Work out the finished part from the listing and answer in its coordinate system (mm). A direction names the side the tool comes from. Coordinates: 2 decimals unless noted, no trailing zeros. Loops run counter-clockwise (first coordinate to the right, second up) from the corner with the lowest first, then second, coordinate; pieces in that order, holes last. Notation, with made-up numbers: (-9.5, 84) -> (4.5, 84) arc R31 cw to (4.5, 115) -> close; hole circle Ø8 at (-4, 51). An arc over 180 degrees is marked (long way). Use a Markdown table: item, result.
from build123d import *

# Parameters (mm, degrees)
SKETCH1_R           = 21.25
SKETCH1_R_2         = 1.5
BOSS_EXTRUDE1_DEPTH = 5
CHAMFER1_SIZE       = 2.5
SKETCH2_R           = 4.75
BOSS_EXTRUDE2_DEPTH = 2


with BuildPart() as part:
    # Sketch1 → Boss-Extrude1 (new body)
    with BuildSketch(Plane(origin=(0, 0, 0), x_dir=(1, 0, 0), z_dir=(0, 1, 0))):
        with Locations(Location((0, 0, 0), (0, 0, 270))):
            Circle(SKETCH1_R)
        with Locations(Location((0, 15.5, 0), (0, 0, 270))):
            Circle(SKETCH1_R_2, mode=Mode.SUBTRACT)
        with Locations(Location((15.5, 0, 0), (0, 0, 270))):
            Circle(SKETCH1_R_2, mode=Mode.SUBTRACT)
        with Locations(Location((0, -15.5, 0), (0, 0, 270))):
            Circle(SKETCH1_R_2, mode=Mode.SUBTRACT)
        with Locations(Location((-15.5, 0, 0), (0, 0, 270))):
            Circle(SKETCH1_R_2, mode=Mode.SUBTRACT)
        with BuildLine():
            Line((-1.532970972, 2.1), (1.532970972, 2.1))
            ThreePointArc((1.532970972, 2.1), (0, -2.6), (-1.532970972, 2.1))
        make_face(mode=Mode.SUBTRACT)
    extrude(amount=BOSS_EXTRUDE1_DEPTH)

    # Chamfer1
    chamfer1_edges = [part.edges().sort_by_distance(p)[0] for p in [
        (0, 5, -21.25),
    ]]
    chamfer(chamfer1_edges, length=CHAMFER1_SIZE)

    # Sketch2 → Boss-Extrude2 (add)
    with BuildSketch(Plane(origin=(0, 5, 0), x_dir=(1, 0, 0), z_dir=(0, 1, 0))):
        with Locations(Location((0, 0, 0), (0, 0, 270))):
            Circle(SKETCH2_R)
        with BuildLine():
            Line((1.532970972, 2.1), (-1.532970972, 2.1))
            ThreePointArc((-1.532970972, 2.1), (0, -2.6), (1.532970972, 2.1))
        make_face(mode=Mode.SUBTRACT)
    extrude(amount=BOSS_EXTRUDE2_DEPTH)


solid = part.part
Q1. Section C-C on y = 4.25 is taken. Determine the outline of the cut face in (x, z), and give its area (3 significant figures).
Solved:
| item | result |
|---|---|
| outline | circle Ø39 at (0, 0); hole circle Ø3 at (-15.5, 0); hole (-1.53, -2.1) -> (1.53, -2.1) arc R2.6 ccw (long way) to start; hole circle Ø3 at (0, -15.5); hole circle Ø3 at (0, 15.5); hole circle Ø3 at (15.5, 0) |
| area | 1,150 mm² |
Q2. For faces 1 (the flat face through (-4, 0, 0)), 2 (the flat face through (0, 3, -2.1)), 3 (the cylindrical face through (-2.89, 5.99, -3.77)), determine the directions among +Z, -Z, +X, -X, +Y, -Y from which every point of the face is accessible in a straight line to the end or side of a thin tool.
Solved:
| item | result |
|---|---|
| face 1 | +Z, -Z, +X, -X, -Y |
| face 2 | +Y, -Y |
| face 3 | +Y |
Q3. Section A-A on y = 1 is taken. Determine the outline of the cut face in (x, z), and give its area (3 significant figures).
Solved:
| item | result |
|---|---|
| outline | circle Ø42.5 at (0, 0); hole circle Ø3 at (-15.5, 0); hole (-1.53, -2.1) -> (1.53, -2.1) arc R2.6 ccw (long way) to start; hole circle Ø3 at (0, -15.5); hole circle Ø3 at (0, 15.5); hole circle Ø3 at (15.5, 0) |
| area | 1,370 mm² |
Q4. Given pin 1 Ø3 at (x, y) = (-3.5, 5.5) entering from +Z; pin 2 Ø4 at (x, z) = (-15.5, 0) entering from +Y; pin 3 Ø0.9 at (x, y) = (0.5, 5) entering from +Z; pin 4 Ø1.8 at (x, z) = (0, -15.5) entering from +Y, each flat-ended and moving along its own axis, determine where each tip first touches the part or whether it passes through.
Solved:
| item | result |
|---|---|
| pin 1 | z = 19.46 |
| pin 2 | y = 5 |
| pin 3 | z = 19.19 |
| pin 4 | through |
Q5. Consider line 1 (X direction, y = 1.25, z = 0); line 2 (X direction, y = 3.25, z = 0); line 3 (Z direction, x = 2, y = 1.5). Determine where each line is inside the solid, lowest interval first. Write a range as [from, to].
Solved:
| item | result |
|---|---|
| line 1 | [-21.25, -17], [-14, -2.6], [2.6, 14], [17, 21.25] |
| line 2 | [-20.5, -17], [-14, -2.6], [2.6, 14], [17, 20.5] |
| line 3 | [-21.16, -1.66], [1.66, 21.16] |
Q6. Section B-B on x = 0 is taken. Determine the outline of the cut face in (y, z).
Solved:
| item | result |
|---|---|
| outline | (0, -21.25) -> (2.5, -21.25) -> (5, -18.75) -> (5, -17) -> (0, -17) -> close; (0, -14) -> (5, -14) -> (5, -4.75) -> (7, -4.75) -> (7, -2.1) -> (0, -2.1) -> close; (0, 2.6) -> (7, 2.6) -> (7, 4.75) -> (5, 4.75) -> (5, 14) -> (0, 14) -> close; (0, 17) -> (5, 17) -> (5, 18.75) -> (2.5, 21.25) -> (0, 21.25) -> close |
Q7. Determine the mould class of faces 4 (the cylindrical face through (16.765, 2.465, 0.806)), 5 (the cylindrical face through (-12.93, 1.232, -16.863)), 6 (the flat face through (-4, 5, 4)) for opening direction Z: pulls with the +Z half, pulls with the -Z half, needs draft (parallel to the pull), parting line crosses it, or undercut.
Solved:
| item | result |
|---|---|
| face 4 | undercut |
| face 5 | parting line crosses it |
| face 6 | needs draft |
